Here's how the part is built. I have some questions about the finished solid (model axes, mm). A direction names the side the tool comes from. Coordinates: 2 decimals unless noted, no trailing zeros. Write each loop counter-clockwise with the first axis right and the second up, starting at its lowest first coordinate (ties: lowest second). Pieces come first, ordered by that corner, then holes. Notation, with made-up numbers: (32.5, 7.5) -> (39.5, 7.5) arc R17 cw to (39.5, 37.5) -> close; hole circle Ø10 at (17, 66.5). An arc over 180 degrees is marked (long way). Put each result on its own line as item: value.
```python
from build123d import *

# Parameters (mm, degrees)
SKETCH1_W           = 25
SKETCH1_H           = 23
BOSS_EXTRUDE1_DEPTH = 1
SKETCH2_W           = 17
SKETCH2_H           = 16
BOSS_EXTRUDE2_DEPTH = 2
SKETCH3_W           = 6.336645523
SKETCH3_H           = 3.765253137
BOSS_EXTRUDE3_DEPTH = 2.5
SKETCH4_W           = 1.193860751
SKETCH4_H           = 2.357109687
BOSS_EXTRUDE4_DEPTH = 1
SKETCH5_W           = 1.2
SKETCH5_H           = 2.357109687
BOSS_EXTRUDE5_DEPTH = 1
SKETCH6_R           = 0.75
BOSS_EXTRUDE6_DEPTH = 1.5
SKETCH7_R           = 0.635
CUT_EXTRUDE1_DEPTH  = 1.5
SKETCH8_W           = 15
SKETCH8_H           = 17.5
BOSS_EXTRUDE7_DEPTH = 2


with BuildPart() as part:
    # Sketch1 → Boss-Extrude1 (new body)
    with BuildSketch(Plane(origin=(0, 0, 0), x_dir=(0, 0, -1), z_dir=(1, 0, 0))):
        with Locations((12.5, -11.5)):
            Rectangle(SKETCH1_W, SKETCH1_H)
    extrude(amount=BOSS_EXTRUDE1_DEPTH)

    # Sketch2 → Boss-Extrude2 (add)
    with BuildSketch(Plane(origin=(1, 0, 0), x_dir=(0, 0, -1), z_dir=(1, 0, 0))):
        with Locations((12.5, -14)):
            Rectangle(SKETCH2_W, SKETCH2_H)
    extrude(amount=BOSS_EXTRUDE2_DEPTH)

    # Sketch3 → Boss-Extrude3 (add)
    with BuildSketch(Plane(origin=(1, 0, 0), x_dir=(0, 0, -1), z_dir=(1, 0, 0))):
        with Locations((8.107204674, -2.95930386)):
            Rectangle(SKETCH3_W, SKETCH3_H)
    extrude(amount=BOSS_EXTRUDE3_DEPTH)

    # Sketch4 → Boss-Extrude4 (add)
    with BuildSketch(Plane(origin=(1, 0, 0), x_dir=(0, 0, -1), z_dir=(1, 0, 0))):
        with Locations((16.433660331, -3.081751116)):
            Rectangle(SKETCH4_W, SKETCH4_H)
        with Locations((13.433660331, -3.081751116)):
            Rectangle(SKETCH4_W, SKETCH4_H)
        with Locations((19.433660331, -3.081751116)):
            Rectangle(SKETCH4_W, SKETCH4_H)
    extrude(amount=BOSS_EXTRUDE4_DEPTH)

    # Sketch5 → Boss-Extrude5 (add)
    with BuildSketch(Plane(origin=(1, 0, 0), x_dir=(0, 0, -1), z_dir=(1, 0, 0))):
        with Locations((22.430590706, -3.081751116)):
            Rectangle(SKETCH5_W, SKETCH5_H)
    extrude(amount=BOSS_EXTRUDE5_DEPTH)

    # Sketch6 → Boss-Extrude6 (add)
    with BuildSketch(Plane(origin=(1, 0, 0), x_dir=(0, 0, -1), z_dir=(1, 0, 0))):
        with Locations((1.5, -2)):
            Circle(SKETCH6_R)
    extrude(amount=BOSS_EXTRUDE6_DEPTH)

    # Sketch7 → Cut-Extrude1 (cut)
    with BuildSketch(Plane(origin=(1, 0, 0), x_dir=(0, 0, -1), z_dir=(1, 0, 0))):
        with Locations((1.5, -4.54)):
            Circle(SKETCH7_R)
        with Locations((1.5, -7.04)):
            Circle(SKETCH7_R)
        with Locations((1.5, -9.54)):
            Circle(SKETCH7_R)
        with Locations((1.5, -12.04)):
            Circle(SKETCH7_R)
        with Locations((1.5, -14.54)):
            Circle(SKETCH7_R)
        with Locations((1.5, -17.04)):
            Circle(SKETCH7_R)
        with Locations((23.5, -21)):
            Circle(SKETCH7_R)
        with Locations((23.5, -18.5)):
            Circle(SKETCH7_R)
        with Locations((23.5, -16)):
            Circle(SKETCH7_R)
        with Locations((23.5, -13.5)):
            Circle(SKETCH7_R)
        with Locations((23.5, -11)):
            Circle(SKETCH7_R)
        with Locations((23.5, -8.5)):
            Circle(SKETCH7_R)
    extrude(amount=-CUT_EXTRUDE1_DEPTH, mode=Mode.SUBTRACT)

    # Sketch8 → Boss-Extrude7 (add)
    with BuildSketch(Plane.ZY):
        with Locations((-12.5, -13.75)):
            Rectangle(SKETCH8_W, SKETCH8_H)
    extrude(amount=BOSS_EXTRUDE7_DEPTH)


solid = part.part
```
Item 1: Imagine slicing it at D-D on y = -13.5. Write out the boundary of the cut face in (x, z) (3 decimals), then the cut area to 3 significant figures.
Output:
outline: (-2, -20) -> (0, -20) -> (0, -22.865) -> (1, -22.865) -> (1, -21) -> (3, -21) -> (3, -4) -> (1, -4) -> (1, 0) -> (0, 0) -> (0, -5) -> (-2, -5) -> close; (0, -25) -> (1, -25) -> (1, -24.135) -> (0, -24.135) -> close
area: 87.7 mm²
Item 2: Imagine slicing it at A-A on z = -1.5. State how many separate pieces and enclosed holes the cut face has, then the cut area to 3 significant figures.
Output:
separate pieces: 7
enclosed holes: 0
area: 17.6 mm²
Item 3: Imagine slicing it at B-B on y = -4.54. Write out the boundary of the cut face in (x, z) (3 decimals).
Output:
outline: (0, -25) -> (1, -25) -> (1, -11.276) -> (3.5, -11.276) -> (3.5, -4.939) -> (1, -4.939) -> (1, -2.135) -> (0, -2.135) -> close; (0, -0.865) -> (1, -0.865) -> (1, 0) -> (0, 0) -> close
Item 4: Which directions (+Z, -Z, +X, -X, +Y, -Y) give clear straight access to the entire face, cutting with the end or side of a thin tool? Please do faces 1 (the flat face through (2, -1.077, -8)), 2 (the flat face through (-1, -14, -5)), 3 (the flat face through (2, -3, -16)), 4 (the flat face through (-1, -22.5, -13)), 5 (the flat face through (1.5, -4.26, -13.4)).
Output:
face 1: +Z, -Z, +X, +Y
face 2: +Z, -X, +Y, -Y
face 3: -Z, +X, +Y
face 4: +Z, -Z, -X, -Y
face 5: -Z, +X
Item 5: If we mould it in two halves opening along Z, with no side actions, what happens to faces 6 (the flat face through (1.5, -4.26, -22.4)), 7 (the cylindrical face through (0.51, -16.24, -24.09)), 8 (the flat face through (2, -14, -4))? For each: released by +Z, released by -Z, zero draft, split by the parting line, or undercut.
Output:
face 6: zero draft
face 7: undercut
face 8: released by +Z
Item 6: For P1, Ø1, axis at x = 2, z = -14.5, coming from the -Y side; P2, Ø0.8, axis at x = 1.5, y = -3, coming from the +Z side; P3, Ø0.6, axis at x = -1, y = -9.5, coming from the +Z side; P4, Ø12, axis at y = -4, z = -12, coming from the +X side, each with a flat end and sliding along its axis, tell me the tip position at first contact or that it passes through.
Output:
P1: stops at y = -22
P2: stops at z = -1.05
P3: stops at z = -5
P4: stops at x = 3.5
Item 7: Please list where these lines run through material, in increasing order: line 1 along Y through (x, z) = (1.05, -11.5); line 2 along X through (y, z) = (-13.25, -21.25); line 3 along Y through (x, z) = (-1.6, -7.75). Write a range as from..to.
Output:
line 1: y = -22..-6
line 2: x = 0..1
line 3: y = -22.5..-5
